Part model, mm, in its own coordinate system. Round coordinates to 2 decimals unless told otherwise and drop trailing zeros. Write each loop counter-clockwise with the first axis right and the second up, starting at its lowest first coordinate (ties: lowest second). Pieces come first, ordered by that corner, then holes.
```python
from build123d import *

# Parameters (mm, degrees)
F1_DEPTH = 5


with BuildPart() as f1:
    # F0 (on Top) → F1 (new body)
    with BuildSketch(Plane.XY):
        with BuildLine():
            Line((0, 2.5), (0, 5))
            ThreePointArc((0, 5), (-5, 0), (0, -5))
            Line((0, -5), (0, -2.5))
            ThreePointArc((0, -2.5), (-2.5, 0), (0, 2.5))
        make_face()
        with BuildLine():
            ThreePointArc((0, -5), (3.535534, -3.535534), (5, 0))
            ThreePointArc((5, 0), (3.535534, 3.535534), (0, 5))
            Line((0, 5), (0, 2.5))
            ThreePointArc((0, 2.5), (1.767767, 1.767767), (2.5, 0))
            ThreePointArc((2.5, 0), (1.767767, -1.767767), (0, -2.5))
            Line((0, -2.5), (0, -5))
        make_face()
        with BuildLine():
            ThreePointArc((0, 5), (3.535534, 3.535534), (5, 0))
            ThreePointArc((5, 0), (3.535534, -3.535534), (0, -5))
            Line((0, -5), (25.098907, -5))
            ThreePointArc((25.098907, -5), (20.098907, 0), (25.098907, 5))
            Line((25.098907, 5), (0, 5))
        make_face()
        with BuildLine():
            Line((25.098907, 2.5), (25.098907, 5))
            ThreePointArc((25.098907, 5), (20.098907, 0), (25.098907, -5))
            Line((25.098907, -5), (25.098907, -2.5))
            ThreePointArc((25.098907, -2.5), (22.598907, 0), (25.098907, 2.5))
        make_face()
        with BuildLine():
            ThreePointArc((30.098907, 0), (28.634441, 3.535534), (25.098907, 5))
            Line((25.098907, 5), (25.098907, 2.5))
            ThreePointArc((25.098907, 2.5), (26.866674, 1.767767), (27.598907, 0))
            ThreePointArc((27.598907, 0), (26.866674, -1.767767), (25.098907, -2.5))
            Line((25.098907, -2.5), (25.098907, -5))
            ThreePointArc((25.098907, -5), (28.634441, -3.535534), (30.098907, 0))
        make_face()
    extrude(amount=F1_DEPTH)


solid = f1.part
```
Q1. Cut at C-C on y = 3.25. Write the cut outline in (x, z), plus the area to 3 significant figures.
Values follow:
outline: (-3.8, 0) - (28.9, 0) - (28.9, 5) - (-3.8, 5) - close
area: 163 mm2
Q2. Drop flat-ended pins along their axis: pin 1 (3 mm diameter, centred on x = 2, y = -3, fed in from -Z); pin 2 (3 mm diameter, centred on y = -2, z = 3.5, fed in from -X); pin 3 (2 mm diameter, centred on y = 2, z = 2.5, fed in from +X). Give the stop position or say it passes through.
Values follow:
pin 1: stops at z = 0
pin 2: stops at x = -4.97
pin 3: stops at x = 30
Q3. Cut at B-B on y = 1.5. Write the cut outline in (x, z).
Values follow:
outline: (-4.77, 0) - (-2, 0) - (-2, 5) - (-4.77, 5) - close; (2, 0) - (23.1, 0) - (23.1, 5) - (2, 5) - close; (27.1, 0) - (29.87, 0) - (29.87, 5) - (27.1, 5) - close
Q4. Wall check: L1, parallel to Y at x = 25, z = 1.05; L2, parallel to X at y = 2, z = 4; L3, parallel to X at y = 0.75, z = 2.7. Give the ranges that are in metal, low to high.
Values follow:
L1: y = -5 to -2.5, 2.5 to 5
L2: x = -4.58 to -1.5, 1.5 to 23.6, 26.6 to 29.68
L3: x = -4.94 to -2.38, 2.38 to 22.71, 27.48 to 30.04
Q5. Cut at A-A on z = 1. Write the cut outline in (x, y), plus the area to 3 significant figures.
Values follow:
outline: (0, -5) - (25.1, -5) arc R5 ccw to (25.1, 5) - (0, 5) arc R5 ccw to start; hole circle Ø5 at (0, 0); hole circle Ø5 at (25.1, 0)
area: 290 mm2
